Input: part model. Units: mm. Frame: model coordinates. Round coordinates to 2 decimals unless told otherwise and drop trailing zeros. Loops run counter-clockwise (first coordinate to the right, second up) from the corner with the lowest first, then second, coordinate; pieces in that order, holes last. Notation, with made-up numbers: (29.25, 37) - (59.25, 37) arc R32 ccw to (59.25, 70) - close; hole circle Ø6 at (68, -5.75). An arc over 180 degrees is marked (long way). One line per question, with ' | ' between items. Start each with the question number.
from build123d import *

# Parameters (mm, degrees)
SKETCH1_W           = 120
SKETCH1_H           = 120
SKETCH1_W_2         = 116.5
SKETCH1_H_2         = 116.5
SKETCH1_R           = 2
BOSS_EXTRUDE1_DEPTH = 4
SKETCH2_W           = 272
SKETCH2_H           = 152
SKETCH2_R           = 1.65
SKETCH2_W_2         = 240
SKETCH2_H_2         = 120
BOSS_EXTRUDE2_DEPTH = 4
FILLET1_R           = 8
SKETCH3_W           = 120
SKETCH3_H           = 86.50757595
CUT_EXTRUDE3_DEPTH  = 211.256985615


with BuildPart() as part:
    # Sketch1 → Boss-Extrude1 (new body)
    with BuildSketch(Plane(origin=(0, 0, 0), x_dir=(1, 0, 0), z_dir=(0, 1, 0))):
        Rectangle(SKETCH1_W, SKETCH1_H)
        Rectangle(SKETCH1_W_2, SKETCH1_H_2, mode=Mode.SUBTRACT)
        with BuildLine():
            Line((-58.25, -58.25), (-28.843326785, -58.25))
            ThreePointArc((-28.843326785, -58.25), (-45.961940777, -45.961940777), (-58.25, -28.843326785))
            Line((-58.25, -28.843326785), (-58.25, -58.25))
        make_face()
        with Locations(Location((-52.5, -52.5, 0), (0, 0, 270))):
            Circle(SKETCH1_R, mode=Mode.SUBTRACT)
        with BuildLine():
            Line((-58.25, 58.25), (-58.25, 28.843326785))
            ThreePointArc((-58.25, 28.843326785), (-45.961940777, 45.961940777), (-28.843326785, 58.25))
            Line((-28.843326785, 58.25), (-58.25, 58.25))
        make_face()
        with Locations(Location((-52.5, 52.5, 0), (0, 0, 270))):
            Circle(SKETCH1_R, mode=Mode.SUBTRACT)
        with BuildLine():
            ThreePointArc((28.843326785, 58.25), (45.961940777, 45.961940777), (58.25, 28.843326785))
            Line((58.25, 28.843326785), (58.25, 58.25))
            Line((58.25, 58.25), (28.843326785, 58.25))
        make_face()
        with Locations(Location((52.5, 52.5, 0), (0, 0, 270))):
            Circle(SKETCH1_R, mode=Mode.SUBTRACT)
        with BuildLine():
            Line((28.843326785, -58.25), (58.25, -58.25))
            Line((58.25, -58.25), (58.25, -28.843326785))
            ThreePointArc((58.25, -28.843326785), (45.961940777, -45.961940777), (28.843326785, -58.25))
        make_face()
        with Locations(Location((52.5, -52.5, 0), (0, 0, 270))):
            Circle(SKETCH1_R, mode=Mode.SUBTRACT)
    boss_extrude1 = extrude(amount=BOSS_EXTRUDE1_DEPTH)

    # Mirror1: Boss-Extrude1 across plane
    add(boss_extrude1.mirror(Plane(origin=(60, 4, 0), x_dir=(0, 0, 1), z_dir=(-1, 0, 0))))

    # Sketch2 → Boss-Extrude2 (add)
    with BuildSketch(Plane(origin=(0, 0, 0), x_dir=(1, 0, 0), z_dir=(0, 1, 0))):
        with Locations((60, 0)):
            Rectangle(SKETCH2_W, SKETCH2_H)
        with Locations(Location((188, 68, 0), (0, 0, 270))):
            Circle(SKETCH2_R, mode=Mode.SUBTRACT)
        with Locations(Location((60, 68, 0), (0, 0, 270))):
            Circle(SKETCH2_R, mode=Mode.SUBTRACT)
        with Locations(Location((-68, 68, 0), (0, 0, 270))):
            Circle(SKETCH2_R, mode=Mode.SUBTRACT)
        with Locations(Location((-68, -68, 0), (0, 0, 90))):
            Circle(SKETCH2_R, mode=Mode.SUBTRACT)
        with Locations(Location((60, -68, 0), (0, 0, 90))):
            Circle(SKETCH2_R, mode=Mode.SUBTRACT)
        with Locations(Location((188, -68, 0), (0, 0, 90))):
            Circle(SKETCH2_R, mode=Mode.SUBTRACT)
        with Locations((60, 0)):
            Rectangle(SKETCH2_W_2, SKETCH2_H_2, mode=Mode.SUBTRACT)
    extrude(amount=BOSS_EXTRUDE2_DEPTH)

    # Fillet1
    fillet1_edges = [part.edges().sort_by_distance(p)[0] for p in [
        (196, 2, -76),
        (-76, 2, -76),
        (-76, 2, 76),
        (196, 2, 76),
    ]]
    fillet(fillet1_edges, radius=FILLET1_R)

    # Sketch3 → Cut-Extrude3 (cut, through all)
    with BuildSketch(Plane(origin=(0, 0, 0), x_dir=(1, 0, 0), z_dir=(0, 1, 0))):
        with Locations((60, 0)):
            Rectangle(SKETCH3_W, SKETCH3_H)
    extrude(amount=CUT_EXTRUDE3_DEPTH, mode=Mode.SUBTRACT)


solid = part.part
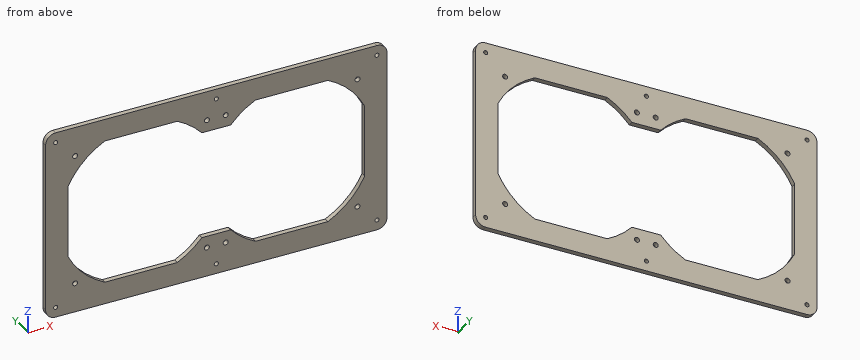
(1) Section C-C, the plane y = 3. Give the number of separate pieces and of enclosed holes in the cut face, plus the area to 3 significant figures.
(2) Section A-A, the plane z = -39. Output: boundary loops of the cut face in (x, y), plus the area to 3 significant figures.
(3) Section B-B, the plane x = -33. Output: boundary loops of the cut face in (y, z), plus the area to 3 significant figures.
(4) Line query: line 1 along Z through (x, y) = (188, 2.75); line 2 along X through (y, z) = (2.7, -68); line 3 along Z through (x, y) = (135.5, 3.15). Output: solid intervals per line, ascending. Write a range as from..to.
(5) Pin query (flat end, axial travel): P1, Ø6.5, axis at x = 172.5, z = -52.5, coming from the +Y side; P2, Ø2.5, axis at x = 52.5, z = -52.5, coming from the +Y side. Return the tip coordinate at first contact, or that it passes through.
Derived:
1) separate pieces: 1 | enclosed holes: 15 | area: 16,100 mm²
2) outline: (-76, 0) - (-52, 0) - (-52, 4) - (-76, 4) - close; (172, 0) - (196, 0) - (196, 4) - (172, 4) - close | area: 192 mm²
3) outline: (0, -76) - (4, -76) - (4, -56) - (0, -56) - close; (0, 56) - (4, 56) - (4, 76) - (0, 76) - close | area: 160 mm²
4) line 1: z = -76..-69.65, -66.35..66.35, 69.65..76 | line 2: x = -76..-69.65, -66.35..58.35, 61.65..186.35, 189.65..196 | line 3: z = -76..-58.25, 58.25..76
5) P1: stops at y = 4 | P2: passes through
